```python
from build123d import *

# Parameters (mm, degrees)
SCHIZZO1_W                   = 121
SCHIZZO1_H                   = 166
ESTRUSIONE_ESTRUSIONE1_DEPTH = 20
RACCORDO1_R                  = 5
TAGLIO_ESTRUSIONE1_DEPTH     = 14.5
SCHIZZO3_R                   = 2.25
TAGLIO_ESTRUSIONE2_DEPTH     = 105.638663982
TAGLIO_ESTRUSIONE3_DEPTH     = 1.5
SCHIZZO5_W                   = 11
SCHIZZO5_H                   = 11
TAGLIO_ESTRUSIONE4_DEPTH     = 3.5
TAGLIO_ESTRUSIONE5_DEPTH     = 3.5
SCHIZZO11_W                  = 8.5
SCHIZZO11_H                  = 17
SCHIZZO11_W_2                = 7
SCHIZZO11_H_2                = 25
TAGLIO_ESTRUSIONE9_DEPTH     = 10
SCHIZZO12_W                  = 16.5
SCHIZZO12_H                  = 73
TAGLIO_ESTRUSIONE10_DEPTH    = 0.5
SCHIZZO13_R                  = 2.5
SCHIZZO13_R_2                = 1.25
SCHIZZO13_R_3                = 1.425
ESTRUSIONE_ESTRUSIONE3_DEPTH = 5
SCHIZZO14_W                  = 8
SCHIZZO14_H                  = 12
TAGLIO_ESTRUSIONE11_DEPTH    = 3
SCHIZZO15_W                  = 4
SCHIZZO15_H                  = 7
TAGLIO_ESTRUSIONE12_DEPTH    = 3
SCHIZZO16_W                  = 4
SCHIZZO16_H                  = 2
ESTRUSIONE_ESTRUSIONE4_DEPTH = 3
SCHIZZO17_W                  = 5
SCHIZZO17_H                  = 9
TAGLIO_ESTRUSIONE13_DEPTH    = 1
SCHIZZO18_W                  = 2.5
SCHIZZO18_H                  = 1.4
ESTRUSIONE_ESTRUSIONE5_DEPTH = 10


with BuildPart() as part:
    # Schizzo1 → Estrusione-Estrusione1 (new body)
    with BuildSketch(Plane.XY):
        Rectangle(SCHIZZO1_W, SCHIZZO1_H)
    extrude(amount=ESTRUSIONE_ESTRUSIONE1_DEPTH)

    # Raccordo1
    raccordo1_edges = [part.edges().sort_by_distance(p)[0] for p in [
        (-60.5, 83, 10),
        (60.5, 83, 10),
        (60.5, -83, 10),
        (-60.5, -83, 10),
    ]]
    fillet(raccordo1_edges, radius=RACCORDO1_R)

    # Schizzo2 → Taglio-Estrusione1 (cut)
    with BuildSketch(Plane(origin=(0, 0, 0), x_dir=(-1, 0, 0), z_dir=(0, 0, -1))):
        Polygon((-51.5, 80), (51.5, 80), (51.5, 74), (57.5, 74), (57.5, -74), (51.5, -74), (51.5, -80), (-51.5, -80), (-51.5, -74), (-57.5, -74), (-57.5, 74), (-51.5, 74), align=None)
    extrude(amount=-TAGLIO_ESTRUSIONE1_DEPTH, mode=Mode.SUBTRACT)

    # Schizzo3 → Taglio-Estrusione2 (cut, through all)
    with BuildSketch(Plane(origin=(0, 0, 0), x_dir=(-1, 0, 0), z_dir=(0, 0, -1))):
        with Locations((-54.5, 77)):
            Circle(SCHIZZO3_R)
        with Locations((54.5, 77)):
            Circle(SCHIZZO3_R)
        with Locations((54.5, -77)):
            Circle(SCHIZZO3_R)
        with Locations((-54.5, -77)):
            Circle(SCHIZZO3_R)
    extrude(amount=-TAGLIO_ESTRUSIONE2_DEPTH, mode=Mode.SUBTRACT)

    # Schizzo4 → Taglio-Estrusione3 (cut)
    with BuildSketch(Plane(origin=(0, 0, 0), x_dir=(-1, 0, 0), z_dir=(0, 0, -1))):
        with BuildLine():
            Line((-55.5, 81.5), (55.5, 81.5))
            ThreePointArc((55.5, 81.5), (57.974873734, 80.474873734), (59, 78))
            Line((59, 78), (59, -78))
            ThreePointArc((59, -78), (57.974873734, -80.474873734), (55.5, -81.5))
            Line((55.5, -81.5), (-55.5, -81.5))
            ThreePointArc((-55.5, -81.5), (-57.974873734, -80.474873734), (-59, -78))
            Line((-59, -78), (-59, 78))
            ThreePointArc((-59, 78), (-57.974873734, 80.474873734), (-55.5, 81.5))
        make_face()
    extrude(amount=-TAGLIO_ESTRUSIONE3_DEPTH, mode=Mode.SUBTRACT)

    # Schizzo5 → Taglio-Estrusione4 (cut)
    with BuildSketch(Plane.XY.offset(20)):
        with Locations((-55, 77.5)):
            Rectangle(SCHIZZO5_W, SCHIZZO5_H)
        with Locations((55, 77.5)):
            Rectangle(SCHIZZO5_W, SCHIZZO5_H)
        with Locations((55, -77.5)):
            Rectangle(SCHIZZO5_W, SCHIZZO5_H)
        with Locations((-55, -77.5)):
            Rectangle(SCHIZZO5_W, SCHIZZO5_H)
    extrude(amount=-TAGLIO_ESTRUSIONE4_DEPTH, mode=Mode.SUBTRACT)

    # Schizzo6 → Taglio-Estrusione5 (cut)
    with BuildSketch(Plane(origin=(0, 0, 14.5), x_dir=(-1, 0, 0), z_dir=(0, 0, -1))):
        Polygon((-57.5, 71), (-48.5, 71), (-48.5, 80), (48.5, 80), (48.5, 71), (57.5, 71), (57.5, -71), (48.5, -71), (48.5, -80), (-48.5, -80), (-48.5, -71), (-57.5, -71), align=None)
    extrude(amount=-TAGLIO_ESTRUSIONE5_DEPTH, mode=Mode.SUBTRACT)

    # Schizzo11 → Taglio-Estrusione9 (cut)
    with BuildSketch(Plane.ZY.offset(-57.5)):
        with Locations((10.25, -13.5)):
            Rectangle(SCHIZZO11_W, SCHIZZO11_H)
        with Locations((11, -49.5)):
            Rectangle(SCHIZZO11_W_2, SCHIZZO11_H_2)
    extrude(amount=-TAGLIO_ESTRUSIONE9_DEPTH, mode=Mode.SUBTRACT)

    # Schizzo12 → Taglio-Estrusione10 (cut)
    with BuildSketch(Plane.ZY.offset(-57.5)):
        with Locations((9.75, -33.5)):
            Rectangle(SCHIZZO12_W, SCHIZZO12_H)
    extrude(amount=-TAGLIO_ESTRUSIONE10_DEPTH, mode=Mode.SUBTRACT)

    # Schizzo13 → Estrusione-Estrusione3 (add)
    # profile 1 of 4: a face of its own
    with BuildSketch(Plane(origin=(0, 0, 18), x_dir=(-1, 0, 0), z_dir=(0, 0, -1))):
        with Locations(Location((54.5, -49.25, 0), (0, 0, 180))):
            Circle(SCHIZZO13_R)
        with Locations((54.5, -49.25)):
            Circle(SCHIZZO13_R_2, mode=Mode.SUBTRACT)
    # profile 2 of 4: a face of its own
    with BuildSketch(Plane(origin=(0, 0, 18), x_dir=(-1, 0, 0), z_dir=(0, 0, -1))):
        with Locations(Location((54.5, -66.75, 0), (0, 0, 180))):
            Circle(SCHIZZO13_R)
        with Locations((54.5, -66.75)):
            Circle(SCHIZZO13_R_2, mode=Mode.SUBTRACT)
    # profile 3 of 4: a face of its own
    with BuildSketch(Plane(origin=(0, 0, 18), x_dir=(-1, 0, 0), z_dir=(0, 0, -1))):
        with Locations(Location((22.8, -64.7, 0), (0, 0, 180))):
            Circle(SCHIZZO13_R)
        with Locations((22.8, -64.7)):
            Circle(SCHIZZO13_R_2, mode=Mode.SUBTRACT)
    # profile 4 of 4: a face of its own
    with BuildSketch(Plane(origin=(0, 0, 18), x_dir=(-1, 0, 0), z_dir=(0, 0, -1))):
        with Locations(Location((22.8, -51.3, 0), (0, 0, 180))):
            Circle(SCHIZZO13_R)
        with Locations((22.8, -51.3)):
            Circle(SCHIZZO13_R_3, mode=Mode.SUBTRACT)
    extrude(amount=ESTRUSIONE_ESTRUSIONE3_DEPTH)

    # Schizzo14 → Taglio-Estrusione11 (cut)
    with BuildSketch(Plane.ZY.offset(60.5)):
        with Locations((10, -58)):
            Rectangle(SCHIZZO14_W, SCHIZZO14_H)
    extrude(amount=-TAGLIO_ESTRUSIONE11_DEPTH, mode=Mode.SUBTRACT)

    # Schizzo15 → Taglio-Estrusione12 (cut)
    with BuildSketch(Plane(origin=(-57.5, 0, 0), x_dir=(0, 0, -1), z_dir=(1, 0, 0))):
        with Locations((-16, 18)):
            Rectangle(SCHIZZO15_W, SCHIZZO15_H)
    extrude(amount=-TAGLIO_ESTRUSIONE12_DEPTH, mode=Mode.SUBTRACT)

    # Schizzo16 → Estrusione-Estrusione4 (add)
    with BuildSketch(Plane(origin=(0, 0, 18), x_dir=(-1, 0, 0), z_dir=(0, 0, -1))):
        with Locations((55.5, 23.8)):
            Rectangle(SCHIZZO16_W, SCHIZZO16_H)
        with Locations((55.5, 12.2)):
            Rectangle(SCHIZZO16_W, SCHIZZO16_H)
    extrude(amount=ESTRUSIONE_ESTRUSIONE4_DEPTH)

    # Schizzo17 → Taglio-Estrusione13 (cut)
    with BuildSketch(Plane.ZY.offset(60.5)):
        with Locations((15.5, 18)):
            Rectangle(SCHIZZO17_W, SCHIZZO17_H)
    extrude(amount=-TAGLIO_ESTRUSIONE13_DEPTH, mode=Mode.SUBTRACT)

    # Schizzo18 → Estrusione-Estrusione5 (add)
    with BuildSketch(Plane(origin=(0, 0, 14.5), x_dir=(-1, 0, 0), z_dir=(0, 0, -1))):
        with Locations((-59.25, -49.5)):
            Rectangle(SCHIZZO18_W, SCHIZZO18_H)
    extrude(amount=ESTRUSIONE_ESTRUSIONE5_DEPTH)


solid = part.part
```
Model file for the job. Use its own axes, mm. A direction names the side the tool comes from. Give positions to 0.01 mm unless a question says otherwise; leave off trailing zeros. Write each loop counter-clockwise with the first axis right and the second up, starting at its lowest first coordinate (ties: lowest second). Pieces come first, ordered by that corner, then holes. Notation, with made-up numbers: (37.5, 20.5) - (50.5, 20.5) arc R23 ccw to (50.5, 36.5) - close; hole circle Ø5 at (-28.75, 60). An arc over 180 degrees is marked (long way). One line per question, with ' | ' between items. Start each with the question number.
(1) Slice it at A-A on z = 10.25. Give the number of separate pieces and of enclosed holes in the cut face, plus the area to 3 significant figures.
(2) Slice it at B-B on x = 19. Write the cut outline in (y, z).
(3) Two-plate mould, pull along Y, no slides. Class faces 4 (the face through (59.07, 81.5, 8.37)), 5 (the face through (-53.35, -64.53, 15.54)), 6 (the face through (56, -79, 16.5)): +Y half, -Y half, draft (parallel to the pull), parting line (faces both ways), or undercut.
(4) Wall check: line 1 along Y through (x, z) = (-54.5, 3.25); line 2 along Y through (x, z) = (-22.8, 16.45) (3 decimals); line 3 along Y through (x, z) = (-11, 16.25). Give the ranges that are in metal, low to high. Write a range as from..to.
(5) Pin check, flat tips, straight feed: P1, Ø5, axis at x = -54.5, y = -77, coming from the -Z side; P2, Ø10, axis at x = -24.5, y = -26.5, coming from the -Z side; P3, Ø3, axis at x = 59.5, z = 9.5, coming from the -Y side. Stop position of each tip, or through.
(6) 3-axis set-ups, long thin cutter, end or side, ignore diameter. For faces 1 (the face through (-21, -51, 13)), 2 (the face through (55, -72, 18)), 3 (the face through (-55, -72, 18)): which of +Z, -Z, +X, -X, +Y, -Y reach the whole face in a straight line?
(7) Slice it at C-C on y = 49. Write the cut outline in (x, z), plus the area to 4 significant figures.
Results below:
1) separate pieces: 4 | enclosed holes: 4 | area: 1,570 mm^2
2) outline: (-83, 0) - (-81.5, 0) - (-81.5, 1.5) - (-80, 1.5) - (-80, 18) - (80, 18) - (80, 1.5) - (81.5, 1.5) - (81.5, 0) - (83, 0) - (83, 20) - (-83, 20) - close
3) face 4: +Y half | face 5: undercut | face 6: draft
4) line 1: -83..-79.25, -74.75..-74, 74..74.75, 79.25..83 | line 2: -83..-80, -67.2..-65.95, -63.45..-62.2, -53.8..-52.725, -49.875..-48.8, 80..83 | line 3: -83..-80, 80..83
5) P1: z = 1.5 | P2: z = 18 | P3: y = -82.33
6) face 1: -Z | face 2: +Z, +X, -Y | face 3: +Z, -X, -Y
7) outline: (-60.5, 0) - (-59, 0) - (-59, 1.5) - (-57.5, 1.5) - (-57.5, 18) - (57.5, 18) - (57.5, 1.5) - (59, 1.5) - (59, 0) - (60.5, 0) - (60.5, 20) - (-60.5, 20) - close | area: 345.5 mm^2
